Work out the finished part from the listing and answer in its coordinate system (mm). A direction names the side the tool comes from. Coordinates: 2 decimals unless noted, no trailing zeros. Write each loop counter-clockwise with the first axis right and the second up, starting at its lowest first coordinate (ties: lowest second). Pieces come first, ordered by that corner, then holes. Notation, with made-up numbers: (80.25, 70) - (94.25, 70) arc R17 cw to (94.25, 76) - close; hole circle Ø8 at (5, 54.25). An arc over 180 degrees is marked (long way). One line per item, written item: value.
```python
from build123d import *

# Parameters (mm, degrees)
BOSS_EXTRUDE1_DEPTH = 12.15
BOSS_EXTRUDE2_DEPTH = 4.35
SKETCH5_R           = 2.425
BOSS_EXTRUDE3_DEPTH = 3.3
SKETCH6_R           = 0.828221189
CUT_EXTRUDE3_DEPTH  = 4
SKETCH8_R           = 1
CUT_EXTRUDE4_DEPTH  = 5
SKETCH9_W           = 2.165756054
SKETCH9_H           = 0.75
SKETCH9_W_2         = 1.729877666
CUT_EXTRUDE5_DEPTH  = 5
SKETCH10_W          = 3.3
SKETCH10_H          = 1.3
BOSS_EXTRUDE6_DEPTH = 27.5


with BuildPart() as part:
    # Sketch1 → Boss-Extrude1 (new body)
    with BuildSketch(Plane.XY):
        Polygon((-11.25, -11.25), (11.25, -11.25), (11.25, 4.75), (16.25, 4.75), (16.25, 7.15), (11.25, 7.15), (11.25, 11.25), (-11.25, 11.25), (-11.25, 7.15), (-16.25, 7.15), (-16.25, 4.75), (-11.25, 4.75), align=None)
    extrude(amount=BOSS_EXTRUDE1_DEPTH)

    # Sketch4 → Boss-Extrude2 (add)
    with BuildSketch(Plane(origin=(0, 11.25, 0), x_dir=(1, 0, 0), z_dir=(0, 1, 0))):
        with BuildLine():
            ThreePointArc((0.175453629, -3.197801543), (-11.25, -6.075), (0.175453629, -8.952198457))
            ThreePointArc((0.175453629, -8.952198457), (4.025, -6.075), (0.175453629, -3.197801543))
        make_face()
    extrude(amount=BOSS_EXTRUDE2_DEPTH)

    # Sketch5 → Boss-Extrude3 (add)
    with BuildSketch(Plane(origin=(0, 15.6, 0), x_dir=(1, 0, 0), z_dir=(0, 1, 0))):
        with Locations(Location((-5.175, -6.075, 0), (0, 0, 270))):
            Circle(SKETCH5_R)
    extrude(amount=BOSS_EXTRUDE3_DEPTH)

    # Sketch6 → Cut-Extrude3 (cut)
    with BuildSketch(Plane(origin=(0, 18.9, 0), x_dir=(1, 0, 0), z_dir=(0, 1, 0))):
        with Locations(Location((-5.175, -6.075, 0), (0, 0, 270))):
            Circle(SKETCH6_R)
    extrude(amount=-CUT_EXTRUDE3_DEPTH, mode=Mode.SUBTRACT)

    # Sketch8 → Cut-Extrude4 (cut)
    with BuildSketch(Plane(origin=(0, 7.15, 0), x_dir=(1, 0, 0), z_dir=(0, 1, 0))):
        with Locations(Location((-14.65, -6.075, 0), (0, 0, 180))):
            Circle(SKETCH8_R)
        with Locations(Location((14.65, -6.075, 0), (0, 0, 180))):
            Circle(SKETCH8_R)
    extrude(amount=-CUT_EXTRUDE4_DEPTH, mode=Mode.SUBTRACT)

    # Sketch9 → Cut-Extrude5 (cut)
    with BuildSketch(Plane(origin=(0, 7.15, 0), x_dir=(1, 0, 0), z_dir=(0, 1, 0))):
        with Locations((-16.153079265, -6.075)):
            Rectangle(SKETCH9_W, SKETCH9_H)
        with Locations((16.036741918, -6.075)):
            Rectangle(SKETCH9_W_2, SKETCH9_H)
    extrude(amount=-CUT_EXTRUDE5_DEPTH, mode=Mode.SUBTRACT)

    # Sketch10 → Boss-Extrude6 (add)
    with BuildSketch(Plane(origin=(11.25, 0, 0), x_dir=(0, 0, -1), z_dir=(1, 0, 0))):
        with Locations((-6.075, -6.6)):
            Rectangle(SKETCH10_W, SKETCH10_H)
    extrude(amount=-BOSS_EXTRUDE6_DEPTH)


solid = part.part
```
Item 1: Determine the mould class of faces 5 (the face through (-5, 14.9, 6)), 6 (the face through (-6.104, 17.227, 8.315)), 7 (the face through (-16.25, 6, 9)), 8 (the face through (0, 0, 0)) for opening direction Z: +Z half, -Z half, draft (parallel to the pull), parting line (faces both ways), or undercut.
Evaluation:
face 5: undercut
face 6: parting line
face 7: draft
face 8: -Z half
Item 2: Section B-B, the plane x = -14.65 is taken. Determine the outline of the cut face in (y, z) (3 decimals), then the cut area to 4 significant figures.
Evaluation:
outline: (-7.25, 4.425) - (-5.95, 4.425) - (-5.95, 7.725) - (-7.25, 7.725) - close; (4.75, 0) - (7.15, 0) - (7.15, 5.075) - (4.75, 5.075) - close; (4.75, 7.075) - (7.15, 7.075) - (7.15, 12.15) - (4.75, 12.15) - close
area: 28.65 mm2
Item 3: Given pin 1 (1.6 mm diameter, centred on x = -14, z = 6.5, fed in from -Y); pin 2 (0.5 mm diameter, centred on x = -5.5, z = 6, fed in from +Y); pin 3 (4 mm diameter, centred on y = 15, z = 6.5, fed in from +X) (3 decimals), each flat-ended and moving along its own axis, determine where each tip first touches the part or whether it passes through.
Evaluation:
pin 1: stops at y = -7.25
pin 2: stops at y = 14.9
pin 3: stops at x = 4.025
Item 4: Consider probe 1 along Z at (x, y) = (-14.65, 6.65) (3 decimals); probe 2 along X at (y, z) = (9, 10.5); probe 3 along Z at (x, y) = (14, 6). Determine where each line is inside the solid, lowest interval first.
Evaluation:
probe 1: z = 0 to 5.075, 7.075 to 12.15
probe 2: x = -11.25 to 11.25
probe 3: z = 0 to 5.32, 6.83 to 12.15
Item 5: Section D-D, the plane x = -10 is taken. Determine the outline of the cut face in (y, z).
Evaluation:
outline: (-11.25, 0) - (11.25, 0) - (11.25, 2.38) - (15.6, 2.38) - (15.6, 9.77) - (11.25, 9.77) - (11.25, 12.15) - (-11.25, 12.15) - close
Item 6: Section A-A, the plane x = 14.65 is taken. Determine the outline of the cut face in (y, z) (3 decimals).
Evaluation:
outline: (4.75, 0) - (7.15, 0) - (7.15, 5.075) - (4.75, 5.075) - close; (4.75, 7.075) - (7.15, 7.075) - (7.15, 12.15) - (4.75, 12.15) - close
Item 7: Section C-C, the plane z = 11.75 is taken. Determine the outline of the cut face in (x, y), then the cut area to 3 significant figures.
Evaluation:
outline: (-16.25, 4.75) - (-11.25, 4.75) - (-11.25, -11.25) - (11.25, -11.25) - (11.25, 4.75) - (16.25, 4.75) - (16.25, 7.15) - (11.25, 7.15) - (11.25, 11.25) - (-3.01, 11.25) - (-3.01, 15.6) - (-7.34, 15.6) - (-7.34, 11.25) - (-11.25, 11.25) - (-11.25, 7.15) - (-16.25, 7.15) - close
area: 549 mm2
Item 8: Which of the six approach directions +Z, -Z, +X, -X, +Y, -Y give full straight-line access (tool end or side, diameter ignored) to faces 1 (the face through (-13, 4.75, 6)), 2 (the face through (-11.246, 13.395, 5.85)), 3 (the face through (-10, 11.25, 11)), 4 (the face through (-14, -7, 4.425))?
Evaluation:
face 1: +Z, -Z, -X
face 2: +Y
face 3: +Z, -X, +Y
face 4: -Z, -X, -Y
